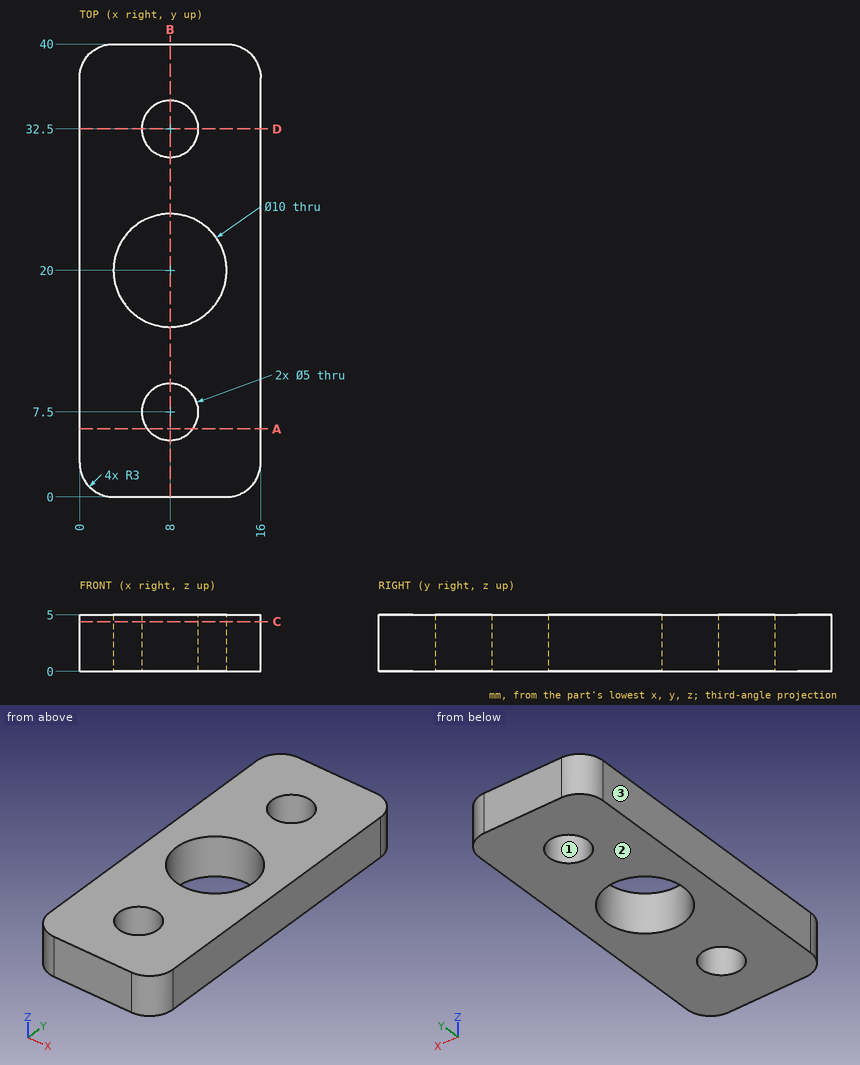
Drawing for the job (mm, zero at the part's lowest x, y, z). Round coordinates to 2 decimals unless told otherwise and drop trailing zeros. Loops run counter-clockwise (first coordinate to the right, second up) from the corner with the lowest first, then second, coordinate; pieces in that order, holes last. Notation, with made-up numbers: (81.25, -16.75) - (95.25, -16.75) arc R18 ccw to (95.25, 4.25) - close; hole circle Ø1 at (67, 89). An arc over 180 degrees is marked (long way). Write each question's results on one line, items separated by ' | '.
(1) Wall check: L1, parallel to Y at x = 8, z = 2.45; L2, parallel to Y at x = 7, z = 1.6; L3, parallel to X at y = 21, z = 2.5. Give the ranges that are in metal, low to high.
Answer below:
L1: y = 0 to 5, 10 to 15, 25 to 30, 35 to 40 | L2: y = 0 to 5.21, 9.79 to 15.1, 24.9 to 30.21, 34.79 to 40 | L3: x = 0 to 3.1, 12.9 to 16
(2) Saw through at D-D, the plane y = 32.5. List the corners of the cut face in (x, z), then the cut area to 3 significant figures.
Answer below:
outline: (0, 0) - (5.5, 0) - (5.5, 5) - (0, 5) - close; (10.5, 0) - (16, 0) - (16, 5) - (10.5, 5) - close | area: 55.0 mm^2
(3) Saw through at A-A, the plane y = 6. List the corners of the cut face in (x, z), then the cut area to 3 significant figures.
Answer below:
outline: (0, 0) - (6, 0) - (6, 5) - (0, 5) - close; (10, 0) - (16, 0) - (16, 5) - (10, 5) - close | area: 60.0 mm^2
(4) Saw through at B-B, the plane x = 8. List the corners of the cut face in (y, z), then the cut area to 3 significant figures.
Answer below:
outline: (0, 0) - (5, 0) - (5, 5) - (0, 5) - close; (10, 0) - (15, 0) - (15, 5) - (10, 5) - close; (25, 0) - (30, 0) - (30, 5) - (25, 5) - close; (35, 0) - (40, 0) - (40, 5) - (35, 5) - close | area: 100 mm^2
(5) Mould opens along X. For the marked faces 1, 2 and 3 say: released by +X, released by -X, zero draft, split by the parting line, or undercut.
Answer below:
face 1: undercut | face 2: zero draft | face 3: released by -X
(6) Saw through at C-C, the plane z = 4.4. List the corners of the cut face in (x, y).
Answer below:
outline: (0, 3) arc R3 ccw to (3, 0) - (13, 0) arc R3 ccw to (16, 3) - (16, 37) arc R3 ccw to (13, 40) - (3, 40) arc R3 ccw to (0, 37) - close; hole circle Ø10 at (8, 20); hole circle Ø5 at (8, 7.5); hole circle Ø5 at (8, 32.5)
